Part model, mm, in its own coordinate system. Coordinates: 2 decimals unless noted, no trailing zeros. Order: outer loops, then holes, each group sorted by start corner. A loop starts at its lowest first (then second) coordinate and runs counter-clockwise, first axis right, second up.
1) Mould opens along X. For faces 1 (the flat face through (163, 137, 4)), 2 (the cylindrical face through (199.241, 181.583, 1.972)) say: +X half, -X half, draft (parallel to the pull), parting line (faces both ways), or undercut.
2) Cut at C-C (z = 3.4). Give the number of separate pieces and of enclosed holes in the cut face, and give its area (3 significant figures).
3) Cut at A-A (x = 200). List the corners of the cut face in (y, z), and give its area (3 significant figures).
4) Cut at B-B (x = 49.5). List the corners of the cut face in (y, z), and give its area (3 significant figures).
5) Wall check: L1, parallel to Y at x = 290, z = 1.8; L2, parallel to Y at x = 89, z = 1.1; L3, parallel to Y at x = 59, z = 1.7. Give the ranges that are in metal, low to high.
```python
from build123d import *

# Parameters (mm, degrees)
SCHIZZO1_W                   = 330
SCHIZZO1_H                   = 270
SCHIZZO1_R                   = 3.5
SCHIZZO1_R_2                 = 1
SCHIZZO1_R_3                 = 3
SCHIZZO1_R_4                 = 4.5
SCHIZZO1_R_5                 = 1.5
SCHIZZO1_W_2                 = 22.7
SCHIZZO1_H_2                 = 10
SCHIZZO1_W_3                 = 65
SCHIZZO1_H_3                 = 7
SCHIZZO1_W_4                 = 4
SCHIZZO1_H_4                 = 20
SCHIZZO1_W_5                 = 5
SCHIZZO1_H_5                 = 15
SCHIZZO1_W_6                 = 12
SCHIZZO1_H_6                 = 5
ESTRUSIONE_ESTRUSIONE1_DEPTH = 4


with BuildPart() as part:
    # Schizzo1 → Estrusione-Estrusione1 (new body)
    with BuildSketch(Plane.XY):
        with Locations((165, 135)):
            Rectangle(SCHIZZO1_W, SCHIZZO1_H)
        with Locations((200, 220)):
            Circle(SCHIZZO1_R, mode=Mode.SUBTRACT)
        with Locations((200, 185)):
            Circle(SCHIZZO1_R, mode=Mode.SUBTRACT)
        with Locations((200, 150)):
            Circle(SCHIZZO1_R, mode=Mode.SUBTRACT)
        with Locations((200, 115)):
            Circle(SCHIZZO1_R, mode=Mode.SUBTRACT)
        with Locations((27, 91)):
            Circle(SCHIZZO1_R_2, mode=Mode.SUBTRACT)
        with Locations((54.5, 91)):
            Circle(SCHIZZO1_R_2, mode=Mode.SUBTRACT)
        with Locations((81, 91)):
            Circle(SCHIZZO1_R_2, mode=Mode.SUBTRACT)
        with Locations((108.5, 91)):
            Circle(SCHIZZO1_R_2, mode=Mode.SUBTRACT)
        with Locations((290, 220)):
            Circle(SCHIZZO1_R_3, mode=Mode.SUBTRACT)
        with Locations((290, 185)):
            Circle(SCHIZZO1_R_3, mode=Mode.SUBTRACT)
        with Locations((290, 150)):
            Circle(SCHIZZO1_R_3, mode=Mode.SUBTRACT)
        with Locations((290, 115)):
            Circle(SCHIZZO1_R_3, mode=Mode.SUBTRACT)
        with Locations((70, 46)):
            Circle(SCHIZZO1_R_4, mode=Mode.SUBTRACT)
        with Locations((59, 46)):
            Circle(SCHIZZO1_R_5, mode=Mode.SUBTRACT)
        with Locations((81, 46)):
            Circle(SCHIZZO1_R_5, mode=Mode.SUBTRACT)
        with Locations((246.35, 185)):
            Rectangle(SCHIZZO1_W_2, SCHIZZO1_H_2, mode=Mode.SUBTRACT)
        with Locations((67.5, 241.5)):
            Rectangle(SCHIZZO1_W_3, SCHIZZO1_H_3, mode=Mode.SUBTRACT)
        with Locations((246.35, 220)):
            Rectangle(SCHIZZO1_W_2, SCHIZZO1_H_2, mode=Mode.SUBTRACT)
        with Locations((246.35, 150)):
            Rectangle(SCHIZZO1_W_2, SCHIZZO1_H_2, mode=Mode.SUBTRACT)
        with Locations((246.35, 115)):
            Rectangle(SCHIZZO1_W_2, SCHIZZO1_H_2, mode=Mode.SUBTRACT)
        with Locations((8, 110)):
            Rectangle(SCHIZZO1_W_4, SCHIZZO1_H_4, mode=Mode.SUBTRACT)
        with Locations((67.5, 124.5)):
            Rectangle(SCHIZZO1_W_3, SCHIZZO1_H_3, mode=Mode.SUBTRACT)
        with Locations((209.563268788, 68.177868744)):
            Rectangle(SCHIZZO1_W_5, SCHIZZO1_H_5, mode=Mode.SUBTRACT)
        with Locations((22.947077827, 12.5)):
            Rectangle(SCHIZZO1_W_6, SCHIZZO1_H_6, mode=Mode.SUBTRACT)
        with Locations((116.687234465, 12.5)):
            Rectangle(SCHIZZO1_W_6, SCHIZZO1_H_6, mode=Mode.SUBTRACT)
        with Locations((209.563268788, 33.177868744)):
            Rectangle(SCHIZZO1_W_5, SCHIZZO1_H_5, mode=Mode.SUBTRACT)
        with Locations((8, 150)):
            Rectangle(SCHIZZO1_W_4, SCHIZZO1_H_4, mode=Mode.SUBTRACT)
        with Locations((8, 70)):
            Rectangle(SCHIZZO1_W_4, SCHIZZO1_H_4, mode=Mode.SUBTRACT)
        with Locations((8, 30)):
            Rectangle(SCHIZZO1_W_4, SCHIZZO1_H_4, mode=Mode.SUBTRACT)
        with Locations((322, 110)):
            Rectangle(SCHIZZO1_W_4, SCHIZZO1_H_4, mode=Mode.SUBTRACT)
        with Locations((322, 150)):
            Rectangle(SCHIZZO1_W_4, SCHIZZO1_H_4, mode=Mode.SUBTRACT)
        with Locations((322, 70)):
            Rectangle(SCHIZZO1_W_4, SCHIZZO1_H_4, mode=Mode.SUBTRACT)
        with Locations((322, 30)):
            Rectangle(SCHIZZO1_W_4, SCHIZZO1_H_4, mode=Mode.SUBTRACT)
    extrude(amount=ESTRUSIONE_ESTRUSIONE1_DEPTH)


solid = part.part
```
Geometry check:
1. face 1: draft
1. face 2: undercut
2. separate pieces: 1
2. enclosed holes: 33
2. area: 86,000 mm2
3. outline: (0, 0) - (111.5, 0) - (111.5, 4) - (0, 4) - close; (118.5, 0) - (146.5, 0) - (146.5, 4) - (118.5, 4) - close; (153.5, 0) - (181.5, 0) - (181.5, 4) - (153.5, 4) - close; (188.5, 0) - (216.5, 0) - (216.5, 4) - (188.5, 4) - close; (223.5, 0) - (270, 0) - (270, 4) - (223.5, 4) - close
3. area: 968 mm2
4. outline: (0, 0) - (121, 0) - (121, 4) - (0, 4) - close; (128, 0) - (238, 0) - (238, 4) - (128, 4) - close; (245, 0) - (270, 0) - (270, 4) - (245, 4) - close
4. area: 1,020 mm2
5. L1: y = 0 to 112, 118 to 147, 153 to 182, 188 to 217, 223 to 270
5. L2: y = 0 to 121, 128 to 238, 245 to 270
5. L3: y = 0 to 44.5, 47.5 to 121, 128 to 238, 245 to 270
